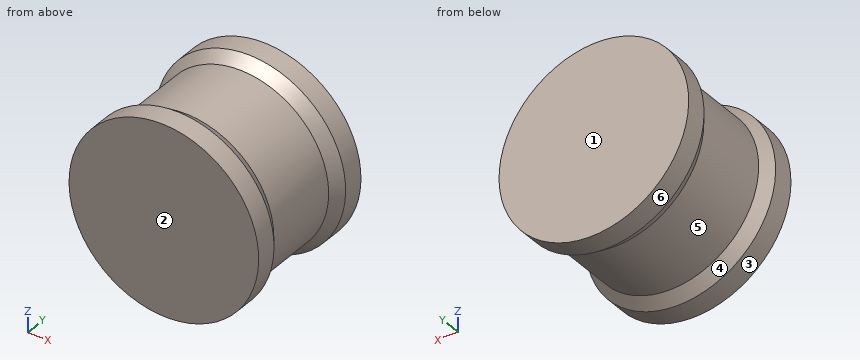
from build123d import *

# Parameters (mm, degrees)
SKETCH2_R           = 20
BOSS_EXTRUDE1_DEPTH = 30


with BuildPart() as part:
    # Sketch2 → Boss-Extrude1 (new body)
    with BuildSketch(Plane(origin=(0, 0, 0), x_dir=(1, 0, 0), z_dir=(0, 1, 0))):
        with Locations(Location((0, 0, 0), (0, 0, 270))):
            Circle(SKETCH2_R)
    extrude(amount=BOSS_EXTRUDE1_DEPTH)

    # Sketch3 → Cut-Revolve1 (revolve, cut)
    with BuildSketch(Plane.XY, mode=Mode.PRIVATE) as cut_revolve1_sk:
        Polygon((-20, 25.507054769), (-18.187675722, 23.049442392), (-18.187675722, 6.950557608), (-20, 4.492945231), align=None)
    revolve(cut_revolve1_sk.sketch.rotate(Axis((0, 30, 0), (0, -1, 0)), 270), axis=Axis((0, 30, 0), (0, -1, 0)), mode=Mode.SUBTRACT)


solid = part.part
Design review of the part built by this model. Coordinates are the model's own, in mm. Face numbers are marked on the shaded views. A direction names the side the tool comes from. Coordinates: 2 decimals unless noted, no trailing zeros. Loops run counter-clockwise (first coordinate to the right, second up) from the corner with the lowest first, then second, coordinate; pieces in that order, holes last. Notation, with made-up numbers: (78.5, 70) - (124.5, 70) arc R15 cw to (124.5, 96) - close; hole circle Ø2 at (-3.75, 57). An arc over 180 degrees is marked (long way). Use CSV: the item, a comma, the result in double quotes. Start each with the question number.
1. To check wall thickness, follow probe 1 along Y at (x, z) = (17.5, 7.5); probe 2 along X at (y, z) = (10.75, -9); probe 3 along Y at (x, z) = (4.5, -18). State the ranges of each line that lie inside material, in increasing order.
2. Add section C-C on y = 10.5. Give the boundary of the cut face in (x, z), plus the area to 3 significant figures.
3. Add section A-A on z = 0. Give the boundary of the cut face in (x, y), plus the area to 3 significant figures.
4. For the marked faces 5 and 6, list the 3-axis set-ups (+Z, -Z, +X, -X, +Y, -Y) from which the entire face can be reached by the end or side of a thin tool; tool diameter is ignored.
5. Mouldability with a two-part tool opening along Y and no side actions: class the marked faces 1, 2, 3 and 4 as released by +Y, released by -Y, zero draft, split by the parting line, or undercut.
6. Add section B-B on x = 0. Give the boundary of the cut face in (y, z).
7. Add section D-D on y = 6.25. Give the boundary of the cut face in (x, z).
8. Clearance check with flat-ended pins moving along their axes: pin 1 (3 mm diameter, centred on y = 13.5, z = -10.5, fed in from -X); pin 2 (3 mm diameter, centred on y = 16, z = 12, fed in from +X); pin 3 (10 mm diameter, centred on y = 10.5, z = 14, fed in from +X); pin 4 (6 mm diameter, centred on x = 1, z = -6.5, fed in from -Y). State where each tip first meets the part, or that it passes through.
Resolved:
1,probe 1,"0 to 5.8, 24.2 to 30"
1,probe 2,"-15.8 to 15.8"
1,probe 3,"0 to 6.45, 23.55 to 30"
2,outline,"circle Ø36.38 at (0, 0)"
2,area,"1,040 mm2"
3,outline,"(-20, 0) - (20, 0) - (20, 4.49) - (18.19, 6.95) - (18.19, 23.05) - (20, 25.51) - (20, 30) - (-20, 30) - (-20, 25.51) - (-18.19, 23.05) - (-18.19, 6.95) - (-20, 4.49) - close"
3,area,"1,130 mm2"
4,face 5,"none"
4,face 6,"+Y, -Y"
5,face 1,"released by +Y"
5,face 2,"released by -Y"
5,face 3,"zero draft"
5,face 4,"undercut"
6,outline,"(0, -20) - (4.49, -20) - (6.95, -18.19) - (23.05, -18.19) - (25.51, -20) - (30, -20) - (30, 20) - (25.51, 20) - (23.05, 18.19) - (6.95, 18.19) - (4.49, 20) - (0, 20) - close"
7,outline,"circle Ø37.41 at (0, 0)"
8,pin 1,"x = -15.8"
8,pin 2,"x = 14.85"
8,pin 3,"x = 15.8"
8,pin 4,"y = 0"
